Geometry check sheet. Reference: the model listing, model coordinates, mm. A direction names the side the tool comes from. Give positions to 0.01 mm unless a question says otherwise; leave off trailing zeros. Write each loop counter-clockwise with the first axis right and the second up, starting at its lowest first coordinate (ties: lowest second). Pieces come first, ordered by that corner, then holes.
(1) Cross-section at D-D (y = -6.25). Record the boundary of the cut face in (x, z) (3 decimals), and give its area (3 significant figures).
(2) Thickness scan on line 1 along Y through (x, z) = (22, 0.5) (3 decimals); line 2 along Z through (x, y) = (37.3, 12.95) (3 decimals); line 3 along Z through (x, y) = (37.3, 14.55). Record the ranges inside material, lowest first.
(3) Cross-section at A-A (x = 21.5). Record the boundary of the cut face in (y, z) (3 decimals).
(4) Tool access check on faces 1 (the flat face through (16, -5.125, 0)), 2 (the flat face through (25, -9, 0)), 3 (the cylindrical face through (12.32, -7.35, 4.88)). Record the directions out of +Z, -Z, +X, -X, +Y, -Y that give a thin tool (end or side, any length) a straight path to the whole face; none if there is none.
(5) Cross-section at B-B (x = 37.3). Record the boundary of the cut face in (y, z) (3 decimals).
(6) Mould release check, pull along Y, two halves, no side actions. Record for faces 4 (the cylindrical face through (36.568, 13.646, -2.987)), 5 (the flat face through (13, -8.425, 0)), 6 (the flat face through (27.24, 7.252, -3.266)): +Y half, -Y half, draft (parallel to the pull), parting line (faces both ways), or undercut.
(7) Depth check by flat-ended pin: P1, Ø1.7, axis at x = 10.5, z = 3.5, coming from the +Y side (3 decimals); P2, Ø2, axis at x = 9.5, z = -0.5, coming from the +Y side (3 decimals); P3, Ø1.2, axis at y = -8, z = 1, coming from the +X side; P4, Ø4, axis at x = 10.5, y = 11, coming from the +Z side. Enter the tip coordinate at first touch or a pass-through.
(8) Cross-section at C-C (z = 0). Record the boundary of the cut face in (x, y) (3 decimals).
```python
from build123d import *

# Parameters (mm, degrees)
BOSS_EXTRUDE1_DEPTH     = 25
CUT_EXTRUDE1_DEPTH      = 28.038606658
CUT_EXTRUDE1_DEPTH_BACK = 28.038606658
SKETCH2_W               = 20
SKETCH2_H               = 10.25
CUT_EXTRUDE2_DEPTH      = 23.496360817
CUT_EXTRUDE2_DEPTH_BACK = 23.496360817
SKETCH3_R               = 2.25
SKETCH5_W               = 11.85
SKETCH5_H               = 4.025
BOSS_EXTRUDE2_DEPTH     = 3
CUT_EXTRUDE3_DEPTH      = 33.370839501
CUT_EXTRUDE3_DEPTH_BACK = 33.370839501
SKETCH6_W               = 16
SKETCH6_H               = 11.85
SKETCH6_R               = 0.75
BOSS_EXTRUDE3_DEPTH     = 3
FILLET1_R               = 2
CHAMFER1_SIZE           = 1.5
CHAMFER2_SIZE           = 0.5


with BuildPart() as part:
    # Sketch1 → Boss-Extrude1 (new body)
    with BuildSketch(Plane(origin=(0, 0, 0), x_dir=(0, 0, -1), z_dir=(1, 0, 0))):
        with BuildLine():
            Line((-4.425, -8.425), (4.425, -8.425))
            ThreePointArc((4.425, -8.425), (4.864339828, -7.364339828), (5.925, -6.925))
            Line((5.925, -6.925), (5.925, 6.925))
            ThreePointArc((5.925, 6.925), (4.864339828, 7.364339828), (4.425, 8.425))
            Line((4.425, 8.425), (-4.425, 8.425))
            ThreePointArc((-4.425, 8.425), (-4.864339828, 7.364339828), (-5.925, 6.925))
            Line((-5.925, 6.925), (-5.925, -6.925))
            ThreePointArc((-5.925, -6.925), (-4.864339828, -7.364339828), (-4.425, -8.425))
        make_face()
    extrude(amount=BOSS_EXTRUDE1_DEPTH)

    # Sketch2 → Cut-Extrude1 (cut, two sides: drawn at the far end of the back side and taken through both)
    with BuildSketch(Plane.XY.offset(-CUT_EXTRUDE1_DEPTH_BACK)):
        with Locations((15, 0)):
            Rectangle(SKETCH2_W, SKETCH2_H)
    extrude(amount=CUT_EXTRUDE1_DEPTH + CUT_EXTRUDE1_DEPTH_BACK, mode=Mode.SUBTRACT)

    # Sketch3 → Cut-Extrude2 (cut, two sides: drawn at the far end of the back side and taken through both)
    with BuildSketch(Plane(origin=(5, 0, 0), x_dir=(0, 0, -1), z_dir=(1, 0, 0)).offset(-CUT_EXTRUDE2_DEPTH_BACK)):
        Circle(SKETCH3_R)
    extrude(amount=CUT_EXTRUDE2_DEPTH + CUT_EXTRUDE2_DEPTH_BACK, mode=Mode.SUBTRACT)

    # Sketch5 → Boss-Extrude2 (add)
    with BuildSketch(Plane(origin=(25, 0, 0), x_dir=(0, 0, -1), z_dir=(1, 0, 0))):
        Polygon((-5.925, 5.125), (5.925, 5.125), (5.925, 9.15), (5.925, 15.125), (-5.925, 15.125), (-5.925, 9.15), align=None)
        with Locations((0, -7.1375)):
            Rectangle(SKETCH5_W, SKETCH5_H)
    extrude(amount=BOSS_EXTRUDE2_DEPTH)

    # Sketch4 → Cut-Extrude3 (cut, two sides: drawn at the far end of the back side and taken through both)
    with BuildSketch(Plane(origin=(28, 0, 0), x_dir=(0, 0, -1), z_dir=(1, 0, 0)).offset(-CUT_EXTRUDE3_DEPTH_BACK)):
        Polygon((-3, 8.925), (3, 8.925), (2, 5.625), (-2, 5.625), align=None)
    extrude(amount=CUT_EXTRUDE3_DEPTH + CUT_EXTRUDE3_DEPTH_BACK, mode=Mode.SUBTRACT)

    # Sketch6 → Boss-Extrude3 (add)
    with BuildSketch(Plane.XZ.offset(-15.125)):
        with Locations((33, 0)):
            Rectangle(SKETCH6_W, SKETCH6_H)
        with Locations(Location((37.3, -3.15, 0), (0, 0, 270))):
            Circle(SKETCH6_R, mode=Mode.SUBTRACT)
        with Locations(Location((37.3, 3.15, 0), (0, 0, 270))):
            Circle(SKETCH6_R, mode=Mode.SUBTRACT)
    extrude(amount=BOSS_EXTRUDE3_DEPTH)

    # Fillet1
    fillet1_edges = [part.edges().sort_by_distance(p)[0] for p in [
        (41, 15.125, 0),
        (33, 15.125, -5.925),
        (33, 15.125, 5.925),
        (26.5, -9.15, 5.925),
        (26.5, -9.15, -5.925),
    ]]
    fillet(fillet1_edges, radius=FILLET1_R)

    # Chamfer1
    chamfer1_edges = [part.edges().sort_by_distance(p)[0] for p in [
        (28, 7.275, -2.5),
        (28, 7.275, 2.5),
    ]]
    chamfer(chamfer1_edges, length=CHAMFER1_SIZE)

    # Chamfer2
    chamfer2_edges = [part.edges().sort_by_distance(p)[0] for p in [
        (0, -8.425, 0),
        (0, 0, 5.925),
        (0, 8.425, 3.636742424),
        (0, 8.425, -3.636742424),
        (0, 0, -5.925),
    ]]
    chamfer(chamfer2_edges, length=CHAMFER2_SIZE)


solid = part.part
```
Reply:
1. outline: (0, -5.425) - (0.5, -5.925) - (28, -5.925) - (28, 5.925) - (0.5, 5.925) - (0, 5.425) - close
1. area: 332 mm2
2. line 1: y = -8.425 to -5.125, 5.125 to 5.625
2. line 2: z = -5.925 to -3.9, -2.4 to 2.4, 3.9 to 5.925
2. line 3: z = -5.33 to -3.9, -2.4 to 2.4, 3.9 to 5.33
3. outline: (-8.425, -4.425) arc R1.5 cw to (-6.925, -5.925) - (-5.125, -5.925) - (-5.125, 5.925) - (-6.925, 5.925) arc R1.5 cw to (-8.425, 4.425) - close; (5.125, -5.925) - (6.925, -5.925) arc R1.5 cw to (8.425, -4.425) - (8.425, -2.848) - (5.625, -2) - (5.625, 2) - (8.425, 2.848) - (8.425, 4.425) arc R1.5 cw to (6.925, 5.925) - (5.125, 5.925) - close
4. face 1: +Z, -Z, +X
4. face 2: -X, -Y
4. face 3: +Z, -X, -Y
5. outline: (12.125, -5.925) - (13.125, -5.925) arc R2 ccw to (15.125, -3.925) - (15.125, -3.9) - (12.125, -3.9) - close; (12.125, -2.4) - (15.125, -2.4) - (15.125, 2.4) - (12.125, 2.4) - close; (12.125, 3.9) - (15.125, 3.9) - (15.125, 3.925) arc R2 ccw to (13.125, 5.925) - (12.125, 5.925) - close
6. face 4: draft
6. face 5: -Y half
6. face 6: undercut
7. P1: stops at y = 8.425
7. P2: stops at y = 5.625
7. P3: stops at x = 28
7. P4: passes through
8. outline: (0, -7.925) - (0.5, -8.425) - (25, -8.425) - (25, -9.15) - (28, -9.15) - (28, -5.125) - (5, -5.125) - (5, -2.25) - (0, -2.25) - close; (0, 2.25) - (5, 2.25) - (5, 5.125) - (28, 5.125) - (28, 5.625) - (0, 5.625) - close; (25, 8.925) - (28, 8.925) - (28, 12.125) - (41, 12.125) - (41, 13.125) arc R2 ccw to (39, 15.125) - (25, 15.125) - close
